Verification items for the finished model (mm, model axes). A direction names the side the tool comes from. Give positions to 0.01 mm unless a question says otherwise; leave off trailing zeros. Loops run counter-clockwise (first coordinate to the right, second up) from the corner with the lowest first, then second, coordinate; pieces in that order, holes last. Notation, with made-up numbers: (9, -25.5) -> (62, -25.5) arc R21 cw to (62, -4.5) -> close; hole circle Ø5 at (35.5, 11). An arc over 180 degrees is marked (long way). Answer in a Markdown table with one row per item. Add a question column.
Q1. Material ranges on probe 1 along X at (y, z) = (-26.5, 5.75); probe 2 along Y at (x, z) = (-155, 6.5); probe 3 along Y at (x, z) = (-50, 2), recorded low to high.
Q2. Section check D-D on x = -78. Enter the section's corners in (y, z), and give its area (3 significant figures).
Q3. Section check B-B on y = -3. Enter the section's corners in (x, z).
Q4. Section check A-A on x = -100. Enter the section's corners in (y, z), and give its area (3 significant figures).
Q5. Release check for a two-part mould opening along Y. For faces 1 (the face through (5, -60, 8)), 2 (the face through (5, -50, 8)), 3 (the face through (-152.691, -10.356, 7.605)), 4 (the face through (-76, -10, 10)) record: pulls with the +Y half, pulls with the -Y half, needs draft (parallel to the pull), parting line crosses it, or undercut.
Q6. Gauge pin test, flat ends, axial feed: P1, Ø3, axis at x = -46, z = 9, coming from the -Y side; P2, Ø4, axis at x = -92.5, z = 12.5, coming from the +Y side; P3, Ø1.5, axis at y = -41.5, z = 3.5, coming from the -X side. Record the tip position at first contact, or that the pin passes through.
Q7. Section check C-C on z = 8.25. Enter the section's corners in (x, y), and give its area (3 significant figures).
Q8. Set-up check for faces 5 (the face through (5, -25, 8)), 6 (the face through (5, -15, 8)), 7 (the face through (0, -76, 7)), 8 (the face through (-25, -10, 13)): record each of +Z, -Z, +X, -X, +Y, -Y from which the full face is reachable in a straight line by a thin tool's end or side.
Autodesk Inventor part; units mm, degrees
ref_plane "YZ Plane" through (0, 0, 0) normal (1, 0, 0) x (0, 1, 0)
ref_plane "XZ Plane" through (0, 0, 0) normal (0, 1, 0) x (-1, 0, 0)
ref_plane "XY Plane" through (0, 0, 0) normal (0, 0, 1) x (1, 0, 0)
sketch "Sketch1" plane through (0, 0, 0) normal (0, 0, 1) x (1, 0, 0)
  circle A0 centre (0, 132.2876) radius 225 construction
  circle A1 centre (0, 132.2876) radius 200 construction
  line L0 (-225, 132.2876) -> (-150, 132.2876) construction
  line L1 (-150, 132.2876) -> (-150, -35.4175) construction
  line L2 (-175, 132.2876) -> (-175, -9.1338) construction
  line L3 (0, 132.2876) -> (0, -92.7124) construction
  line L4 (-150, 0) -> (0, 0)
  line L5 (-175, -9.1338) -> (-175, 0)
  line L6 (0, 0) -> (0, -92.7124)
  arc A2 (-175, -9.1338) -> (0, -92.7124) centre (0, 132.2876) ccw
  line L7 (-167.5, 0) -> (-167.5, 10)
  line L8 (-167.5, 10) -> (-157.5, 10)
  line L9 (-157.5, 10) -> (-157.5, 0)
  line L10 (-175, 0) -> (-167.5, 0)
  line L11 (-157.5, 0) -> (-150, 0)
  dimension "d0" = 450
  dimension "d1" = 25
  dimension "d2" = 75
  dimension "d3" = 25
  dimension "d14" = 10
  dimension "d15" = 10
  dimension "d16" = 90
  dimension "d17" = 7.5
extrude "Extrusion1" add sketch "Sketch1" along normal blind 15
sketch "Sketch2" plane through (0, 0, 15) normal (0, 0, 1) x (1, 0, 0)
  line L0 (10, -15) -> (0, -15)
  line L1 (0, -15) -> (0, -25)
  line L2 (0, -25) -> (10, -25)
  line L3 (10, -25) -> (10, -15)
  line L4 (10, -50) -> (0, -50)
  line L5 (0, -50) -> (0, -60)
  line L6 (0, -60) -> (10, -60)
  line L7 (10, -60) -> (10, -50)
  line L8 (0, 0) -> (0, -95.6231) construction
  line L9 (0, -92.7124) -> (0, 0) construction
  dimension "d6" = 10
  dimension "d7" = 10
  dimension "d8" = 10
  dimension "d9" = 10
  dimension "d10" = 15
  dimension "d11" = 25
extrude "Extrusion2" add sketch "Sketch2" against normal blind 15
sketch "Sketch3" plane through (0, 0, 15) normal (0, 0, 1) x (1, 0, 0)
  line L0 (-25, 0) -> (-125, 0) construction
  line L1 (-125, 0) -> (-125, -20) construction
  line L2 (-125, -20) -> (-25, -20) construction
  line L3 (-25, -20) -> (-25, 0) construction
  line L4 (0, 0) -> (-157.5, 0) construction
  circle A0 centre (-100, -10) radius 2.5
  circle A1 centre (-50, -10) radius 2.5
  dimension "d18" = 100
  dimension "d19" = 20
  dimension "d20" = 25
  dimension "d21" = 5
  dimension "d22" = 5
  dimension "d23" = 25
  dimension "d24" = 25
extrude "Extrusion3" cut sketch "Sketch3" against normal through all
thread "Thread1"
thread "Thread2"
sketch "Sketch5" plane through (0, 0, 15) normal (0, 0, 1) x (1, 0, 0)
  line L0 (-125, 0) -> (-25, 0)
  line L1 (-25, 0) -> (-25, -20)
  line L2 (-25, -20) -> (-125, -20)
  line L3 (-125, -20) -> (-125, 0)
  point P0 (0, 0)
  dimension "d31" = 100
  dimension "d32" = 20
  dimension "d33" = 25
extrude "Extrusion4" cut sketch "Sketch5" against normal blind 5
sketch "Sketch6" plane through (0, 0, 15) normal (0, 0, 1) x (1, 0, 0)
  circle A0 centre (0, 132.2876) radius 225 construction
  arc A1 (-175, -9.1338) -> (0, -92.7124) centre (0, 132.2876) ccw construction
  circle A2 centre (0, 132.2876) radius 210 construction
  circle A3 centre (-155, -9.3987) radius 2.5
  circle A4 centre (-144.4906, -20.1016) radius 2.5
  line L0 (-175, 0) -> (-175, -9.1338)
  point P0 (0, 0)
  dimension "d36" = 450
  dimension "d37" = 15
  dimension "d38" = 5
  dimension "d39" = 5
  dimension "d40" = 15
  dimension "d41" = 20
extrude "Extrusion5" cut sketch "Sketch6" against normal through all
thread "Thread3"
thread "Thread4"
sketch "Sketch7" plane through (0, 0, 15) normal (0, 0, 1) x (1, 0, 0)
  circle A0 centre (-84.0912, -25.1338) radius 2.5
  circle A1 centre (-69.0912, -25.1338) radius 2.5
  line L0 (-125, 0) -> (-25, 0)
  line L1 (-175, 0) -> (-175, -9.1338) construction
  line L2 (-175, -9.1338) -> (22.4277, -9.1338) construction
  point P0 (0, 0)
  dimension "d48" = 5
  dimension "d49" = 5
  dimension "d50" = 69.0912
  dimension "d51" = 15
  dimension "d53" = 16
extrude "Extrusion6" cut sketch "Sketch7" against normal through all
thread "Thread5"
thread "Thread6"
properties part number "CP004" material "ABS Plastic"
Taken from the geometry:
| question | item | result |
|---|---|---|
| 1 | probe 1 | x = -159.41 to -86.18, -82 to -71.18, -67 to 0 |
| 1 | probe 2 | y = -30.81 to -11.9, -6.9 to 0 |
| 1 | probe 3 | y = -87.09 to -12.5, -7.5 to 0 |
| 2 | outline | (-78.76, 0) -> (0, 0) -> (0, 10) -> (-20, 10) -> (-20, 15) -> (-78.76, 15) -> close |
| 2 | area | 1,080 mm² |
| 3 | outline | (-175, 0) -> (0, 0) -> (0, 15) -> (-25, 15) -> (-25, 10) -> (-125, 10) -> (-125, 15) -> (-175, 15) -> close |
| 4 | outline | (-69.27, 0) -> (-12.5, 0) -> (-12.5, 10) -> (-20, 10) -> (-20, 15) -> (-69.27, 15) -> close; (-7.5, 0) -> (0, 0) -> (0, 10) -> (-7.5, 10) -> close |
| 4 | area | 889 mm² |
| 5 | face 1 | pulls with the -Y half |
| 5 | face 2 | undercut |
| 5 | face 3 | undercut |
| 5 | face 4 | needs draft |
| 6 | P1 | stops at y = -88.27 |
| 6 | P2 | stops at y = -20 |
| 6 | P3 | stops at x = -143.82 |
| 7 | outline | (-175, -9.13) arc R225 ccw to (0, -92.71) -> (0, -60) -> (10, -60) -> (10, -50) -> (0, -50) -> (0, -25) -> (10, -25) -> (10, -15) -> (0, -15) -> (0, 0) -> (-157.5, 0) -> (-157.5, 10) -> (-167.5, 10) -> (-167.5, 0) -> (-175, 0) -> close; hole circle Ø5 at (-155, -9.4); hole circle Ø5 at (-144.49, -20.1); hole circle Ø5 at (-100, -10); hole circle Ø5 at (-84.09, -25.13); hole circle Ø5 at (-69.09, -25.13); hole circle Ø5 at (-50, -10) |
| 7 | area | 12,000 mm² |
| 8 | face 5 | +Z, -Z, +X |
| 8 | face 6 | +Z, -Z, +X, +Y |
| 8 | face 7 | +Z, -Z, +X, -Y |
| 8 | face 8 | +Z, +Y |
